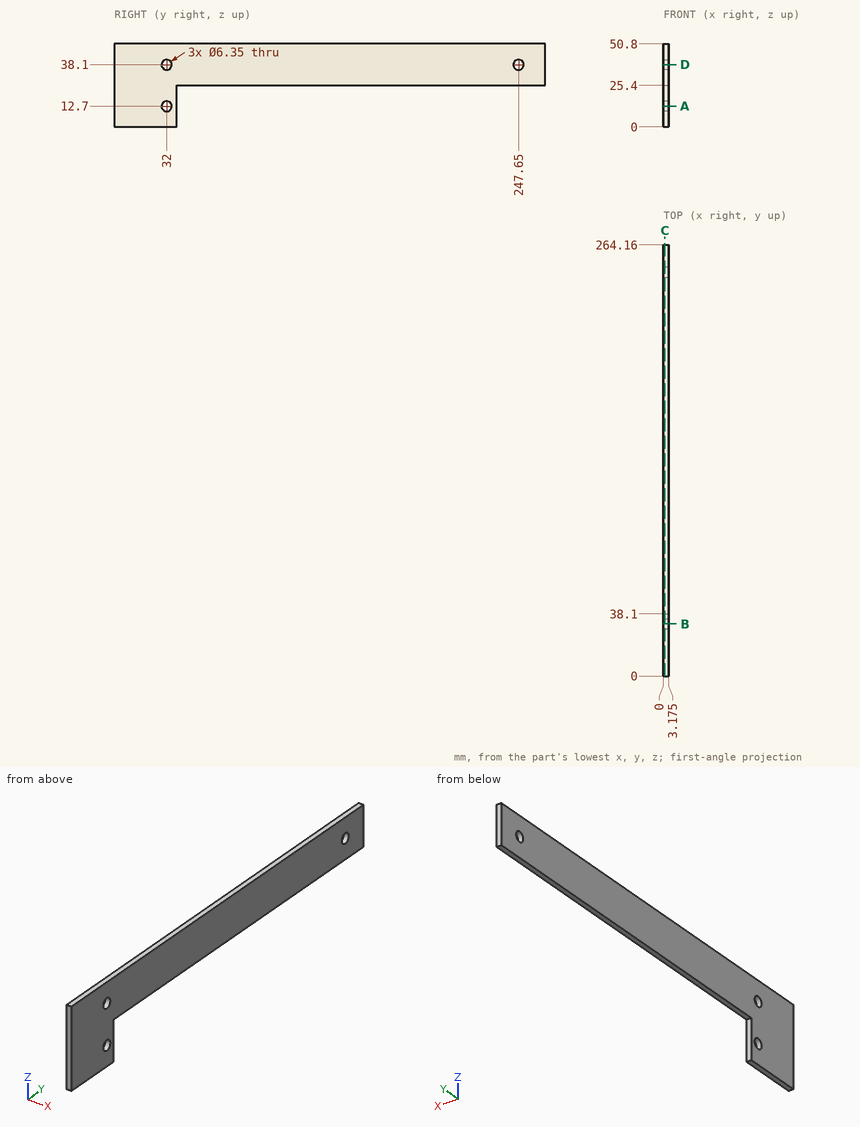
Print and shaded views of the part. All mm, measured from the part's lowest x, y and z. Coordinates: 2 decimals unless noted, no trailing zeros. Order: outer loops, then holes, each group sorted by start corner. A loop starts at its lowest first (then second) coordinate and runs counter-clockwise, first axis right, second up. Notation, with made-up numbers: M 48,-35 L 90,-35 A23 ccw 90,-21 Z; hole C 46.5,-39 d5. An arc over 180 degrees is marked long. Answer as CSV lines item,"result".
1) Cut at D-D (z = 38.1). List the corners of the cut face in (x, y) (3 decimals), then the cut area to 3 significant figures.
Verdict:
outline,"M 0,0 L 3.175,0 L 3.175,28.825 L 0,28.825 Z; M 0,35.175 L 3.175,35.175 L 3.175,244.475 L 0,244.475 Z; M 0,250.825 L 3.175,250.825 L 3.175,264.16 L 0,264.16 Z"
area,"798 mm2"
2) Cut at C-C (x = 0.8). List the corners of the cut face in (y, z) (3 decimals).
Verdict:
outline,"M 0,0 L 38.1,0 L 38.1,25.4 L 264.16,25.4 L 264.16,50.8 L 0,50.8 Z; hole C 32,12.7 d6.35; hole C 32,38.1 d6.35; hole C 247.65,38.1 d6.35"
3) Cut at A-A (z = 12.7). List the corners of the cut face in (x, y) (3 decimals).
Verdict:
outline,"M 0,0 L 3.175,0 L 3.175,28.825 L 0,28.825 Z; M 0,35.175 L 3.175,35.175 L 3.175,38.1 L 0,38.1 Z"
4) Drill centre lines: L1, parallel to Y at x = 1.85, z = 38.1 (3 decimals); L2, parallel to Y at x = 1.2, z = 12.7 (3 decimals); L3, parallel to Z at x = 2, y = 247.65 (3 decimals). Where is each one in solid material? Low to high. Write a range as from..to.
Verdict:
L1,"0..28.825, 35.175..244.475, 250.825..264.16"
L2,"0..28.825, 35.175..38.1"
L3,"25.4..34.925, 41.275..50.8"
5) Cut at B-B (y = 32). List the corners of the cut face in (x, z) (3 decimals).
Verdict:
outline,"M 0,0 L 3.175,0 L 3.175,9.525 L 0,9.525 Z; M 0,15.875 L 3.175,15.875 L 3.175,34.925 L 0,34.925 Z; M 0,41.275 L 3.175,41.275 L 3.175,50.8 L 0,50.8 Z"
6) Flat gauge pins, fed straight in: P1, Ø6, axis at y = 51, z = 34, coming from the -X side; P2, Ø1, axis at x = 2, z = 8, coming from the +Y side; P3, Ø5, axis at y = 32, z = 38.1, coming from the +X side. Where does each tip first touch, or does it go through?
Verdict:
P1,"x = 0"
P2,"y = 38.1"
P3,"through"
